Check sheet for the modelled part. Datum: model origin and axes. Units: mm. Round coordinates to 2 decimals unless told otherwise and drop trailing zeros. Write each loop counter-clockwise with the first axis right and the second up, starting at its lowest first coordinate (ties: lowest second). Pieces come first, ordered by that corner, then holes.
Item 1: Cross-section at C-C on z = 15. Enter the section's corners in (x, y).
Item 2: Cross-section at B-B on z = -33.5. Enter the section's corners in (x, y), plus the area to 3 significant figures.
Item 3: Go/stop test with flat-tipped pins: pin 1 Ø0.9 at (y, z) = (1.5, 6.5) entering from -X; pin 2 Ø1 at (y, z) = (1.5, 11) entering from +X. Record where each tip stops, or that it passes through.
Item 4: Material ranges on line 1 (X direction, y = 1.85, z = -36); line 2 (Z direction, x = -36.5, y = 2.3); line 3 (X direction, y = 1.25, z = -14), recorded low to high.
Item 5: Cross-section at D-D on x = 18.5. Enter the section's corners in (y, z).
Item 6: Cross-section at A-A on x = -37.5. Enter the section's corners in (y, z), plus the area to 3 significant figures.
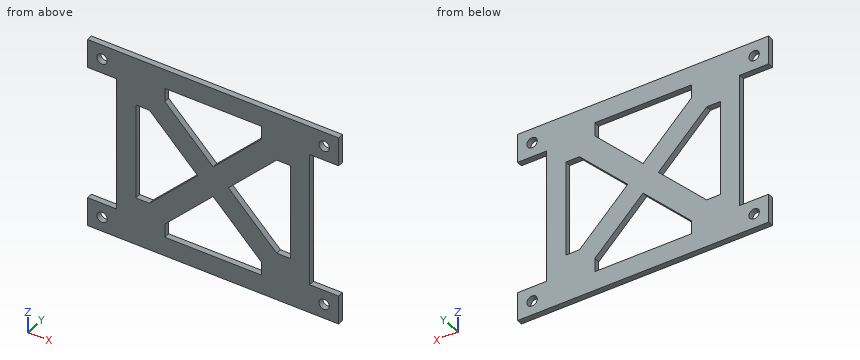
from build123d import *

# Parameters (mm, degrees)
SKETCH2_R           = 2.7
BOSS_EXTRUDE2_DEPTH = 3


with BuildPart() as part:
    # Sketch2 → Boss-Extrude2 (new body)
    with BuildSketch(Plane(origin=(0, 0, 0), x_dir=(1, 0, 0), z_dir=(0, 1, 0))):
        Polygon((50.359735974, 46.638609582), (-49.640264026, 46.638609582), (-64.640264026, 46.638609582), (-64.640264026, 31.638609582), (-49.640264026, 31.638609582), (-49.640264026, -38.361390418), (-64.640264026, -38.361390418), (-64.640264026, -53.361390418), (-49.640264026, -53.361390418), (50.359735974, -53.361390418), (65.359735974, -53.361390418), (65.359735974, -38.361390418), (50.359735974, -38.361390418), (50.359735974, 31.638609582), (65.359735974, 31.638609582), (65.359735974, 46.638609582), align=None)
        with Locations((-57.140264026, -45.861390418)):
            Circle(SKETCH2_R, mode=Mode.SUBTRACT)
        Polygon((25.359735974, -43.361390418), (-24.640264026, -43.361390418), (-24.640264026, -36.290322606), (0.359735974, -11.290322606), (25.359735974, -36.290322606), align=None, mode=Mode.SUBTRACT)
        with Locations((57.859735974, -45.861390418)):
            Circle(SKETCH2_R, mode=Mode.SUBTRACT)
        Polygon((-39.640264026, -28.361390418), (-39.640264026, 21.638609582), (-32.569196215, 21.638609582), (-7.569196215, -3.361390418), (-32.569196215, -28.361390418), align=None, mode=Mode.SUBTRACT)
        Polygon((-24.640264026, 29.56754177), (-24.640264026, 36.638609582), (25.359735974, 36.638609582), (25.359735974, 29.56754177), (0.359735974, 4.56754177), align=None, mode=Mode.SUBTRACT)
        with Locations((-57.140264026, 39.138609582)):
            Circle(SKETCH2_R, mode=Mode.SUBTRACT)
        Polygon((33.288668162, 21.638609582), (40.359735974, 21.638609582), (40.359735974, -28.361390418), (33.288668162, -28.361390418), (8.288668162, -3.361390418), align=None, mode=Mode.SUBTRACT)
        with Locations((57.859735974, 39.138609582)):
            Circle(SKETCH2_R, mode=Mode.SUBTRACT)
    extrude(amount=BOSS_EXTRUDE2_DEPTH)


solid = part.part
Response values:
1. outline: (-49.64, 0) - (-39.64, 0) - (-39.64, 3) - (-49.64, 3) - close; (-19.21, 0) - (-3.35, 0) - (-3.35, 3) - (-19.21, 3) - close; (4.07, 0) - (19.93, 0) - (19.93, 3) - (4.07, 3) - close; (40.36, 0) - (50.36, 0) - (50.36, 3) - (40.36, 3) - close
2. outline: (-64.64, 0) - (-24.64, 0) - (-24.64, 3) - (-64.64, 3) - close; (25.36, 0) - (65.36, 0) - (65.36, 3) - (25.36, 3) - close
2. area: 240 mm2
3. pin 1: stops at x = -49.64
3. pin 2: stops at x = 50.36
4. line 1: x = -64.64 to -24.64, 25.36 to 65.36
4. line 2: z = -46.64 to -21.64, 28.36 to 53.36
4. line 3: x = -49.64 to -39.64, -24.93 to -9.07, 9.79 to 25.65, 40.36 to 50.36
5. outline: (0, -46.64) - (3, -46.64) - (3, -36.64) - (0, -36.64) - close; (0, -22.71) - (3, -22.71) - (3, -6.85) - (0, -6.85) - close; (0, 13.57) - (3, 13.57) - (3, 29.43) - (0, 29.43) - close; (0, 43.36) - (3, 43.36) - (3, 53.36) - (0, 53.36) - close
6. outline: (0, -46.64) - (3, -46.64) - (3, -21.64) - (0, -21.64) - close; (0, 28.36) - (3, 28.36) - (3, 53.36) - (0, 53.36) - close
6. area: 150 mm2
